Autodesk Inventor part; units mm, degrees
ref_plane "YZ Plane" through (0, 0, 0) normal (1, 0, 0) x (0, 1, 0)
ref_plane "XZ Plane" through (0, 0, 0) normal (0, 1, 0) x (-1, 0, 0)
ref_plane "XY Plane" through (0, 0, 0) normal (0, 0, 1) x (1, 0, 0)
sketch "Sketch1" plane through (0, 0, 0) normal (0, 0, 1) x (1, 0, 0)
  line L0 (0, 0) -> (1219.2, 0)
  line L1 (1219.2, 0) -> (1219.2, 609.6)
  line L2 (1219.2, 609.6) -> (0, 609.6)
  line L3 (0, 609.6) -> (0, 0)
  line L4 (658.7784, 301.1028) -> (658.7784, 401.1028)
  line L5 (658.7784, 401.1028) -> (558.7784, 401.1028)
  line L6 (558.7784, 401.1028) -> (558.7784, 201.1028)
  line L7 (558.7784, 201.1028) -> (658.7784, 201.1028)
  line L8 (658.7784, 201.1028) -> (658.7784, 301.1028)
  dimension "d0" = 1219.2
  dimension "d1" = 609.6
  dimension "d4" = 100
  dimension "d5" = 100
  dimension "d6" = 200
  dimension "d7" = 100
extrude "Extrusion1" add sketch "Sketch1" along normal blind 15.875
sketch "Sketch2" plane through (0, 0, 15.875) normal (0, 0, 1) x (1, 0, 0)
  line L0 (658.7784, 201.1028) -> (558.7784, 201.1028)
  line L1 (558.7784, 201.1028) -> (558.7784, 401.1028)
  line L2 (558.7784, 401.1028) -> (658.7784, 401.1028)
  line L3 (658.7784, 401.1028) -> (658.7784, 201.1028)
  line L4 (0, 0) -> (1219.2, 0)
  line L5 (1219.2, 0) -> (1219.2, 609.6)
  line L6 (1219.2, 609.6) -> (0, 609.6)
  line L7 (0, 609.6) -> (0, 0)
sketch "Sketch3" plane through (0, 0, 15.875) normal (0, 0, 1) x (1, 0, 0)
  line L0 (0, 0) -> (859.6758, 0)
  line L1 (0, 0) -> (1219.2, 0)
  line L2 (1219.2, 609.6) -> (0, 609.6)
  line L3 (859.6758, 0) -> (961.2758, 0) construction
  point P0 (859.6758, 101.6)
  point P1 (859.6758, 203.2)
  point P2 (859.6758, 304.8)
  point P3 (859.6758, 355.6)
  point P4 (859.6758, 406.4)
  point P5 (859.6758, 457.2)
  point P6 (859.6758, 508)
  point P7 (859.6758, 558.8)
hole "Hole1" at (859.6758, 101.6, 15.875) at (859.6758, 203.2, 15.875) at (859.6758, 304.8, 15.875) at (859.6758, 355.6, 15.875) at (859.6758, 406.4, 15.875) at (859.6758, 457.2, 15.875) at (859.6758, 508, 15.875) at (859.6758, 558.8, 15.875) direction (0, 0, -1) diameter 3.175 end through all
properties part number "model 2 upper comp front window"
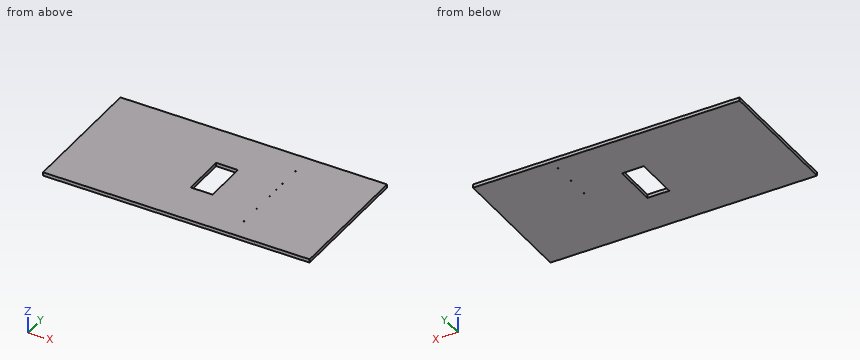
Read the model definition and answer for the solid it produces. Units are mm, in the model's axes. Round coordinates to 2 decimals unless told otherwise and drop trailing zeros. Order: outer loops, then holes, each group sorted by start corner. A loop starts at its lowest first (then second) coordinate and runs counter-clockwise, first axis right, second up.
1) Straight lines are drawn through the part: L1, parallel to X at y = 355.6, z = 11.5; L2, parallel to X at y = 357.5, z = 7.5; L3, parallel to Y at x = 657.5, z = 14. For each, find the intervals that lie inside material, in ascending order.
2) The part is cut by section A-A on y = 229. Write down the section's boundary in (x, z) (3 decimals).
3) The part is cut by section B-B on z = 3. Give the number of separate pieces and of enclosed holes in the cut face, plus the area to 3 significant figures.
Resolved:
1. L1: x = 0 to 558.78, 658.78 to 858.09, 861.26 to 1219.2
1. L2: x = 0 to 558.78, 658.78 to 1219.2
1. L3: y = 0 to 201.1, 401.1 to 609.6
2. outline: (0, 0) - (558.778, 0) - (558.778, 15.875) - (0, 15.875) - close; (658.778, 0) - (1219.2, 0) - (1219.2, 15.875) - (658.778, 15.875) - close
3. separate pieces: 1
3. enclosed holes: 9
3. area: 723,000 mm2
